Read the model definition and answer for the solid it produces. Units are mm, in the model's axes. A direction names the side the tool comes from. Coordinates: 2 decimals unless noted, no trailing zeros. Write each loop counter-clockwise with the first axis right and the second up, starting at its lowest first coordinate (ties: lowest second). Pieces come first, ordered by that corner, then holes. Notation, with made-up numbers: (-1.5, -1) - (51.5, -1) arc R18 cw to (51.5, 29) - close; hole circle Ø11 at (84.5, 48.5). An arc over 180 degrees is marked (long way). Return JSON: item names as keys, results as strings.
```python
from build123d import *

# Parameters (mm, degrees)
BOSS_EXTRUDE1_DEPTH = 34
CUT_EXTRUDE2_START  = -2.320517
SKETCH3_R           = 1.1
CUT_EXTRUDE2_DEPTH  = 2.320517
SKETCH4_R           = 2
CUT_EXTRUDE3_DEPTH  = 1
FILLET1_R           = 2


with BuildPart() as part:
    # Sketch1 → Boss-Extrude1 (new body)
    with BuildSketch(Plane.XY):
        with BuildLine():
            Line((0.25, 38.599190406), (0.25, 41.099190406))
            Line((0.25, 41.099190406), (8.207138981, 40.272184219))
            ThreePointArc((8.207138981, 40.272184219), (8.347930101, 39.521941532), (8.972631806, 39.083268523))
            ThreePointArc((8.972631806, 39.083268523), (0, -40.1), (-8.972631806, 39.083268523))
            ThreePointArc((-8.972631806, 39.083268523), (-8.347930101, 39.521941532), (-8.207138981, 40.272184219))
            Line((-8.207138981, 40.272184219), (-0.25, 41.099190406))
            Line((-0.25, 41.099190406), (-0.25, 38.599190406))
            ThreePointArc((-0.25, 38.599190406), (0, -38.6), (0.25, 38.599190406))
        make_face()
    extrude(amount=BOSS_EXTRUDE1_DEPTH)

    # Sketch3 → Cut-Extrude2 (cut)
    with BuildSketch(Plane(origin=(-4.228569491, 40.685687313, 0), x_dir=(0.994642373, 0.103375773, 0), z_dir=(-0.103375773, 0.994642373, 0)).offset(CUT_EXTRUDE2_START)):
        with Locations((0, -4)):
            Circle(SKETCH3_R)
        with Locations((0, -30)):
            Circle(SKETCH3_R)
    cut_extrude2 = extrude(amount=CUT_EXTRUDE2_DEPTH, mode=Mode.SUBTRACT)

    # Sketch4 → Cut-Extrude3 (cut)
    with BuildSketch(Plane(origin=(-4.228569491, 40.685687313, 0), x_dir=(0.994642373, 0.103375773, 0), z_dir=(-0.103375773, 0.994642373, 0))):
        with Locations((0, -4)):
            Circle(SKETCH4_R)
        with Locations((0, -30)):
            Circle(SKETCH4_R)
    cut_extrude3 = extrude(amount=-CUT_EXTRUDE3_DEPTH, mode=Mode.SUBTRACT)

    # Mirror3: Cut-Extrude2, Cut-Extrude3 across plane
    add(cut_extrude2.mirror(Plane(origin=(0, 0, 0), x_dir=(0, 0, 1), z_dir=(1, 0, 0))), mode=Mode.SUBTRACT)
    add(cut_extrude3.mirror(Plane(origin=(0, 0, 0), x_dir=(0, 0, 1), z_dir=(1, 0, 0))), mode=Mode.SUBTRACT)

    # Fillet1
    fillet1_edges = [part.edges().sort_by_distance(p)[0] for p in [
        (-0.25, 39.849190406, 0),
        (0.25, 39.849190406, 34),
        (0.25, 39.849190406, 0),
        (-0.25, 39.849190406, 34),
    ]]
    fillet(fillet1_edges, radius=FILLET1_R)


solid = part.part
```
(1) A cutting plane is placed at B-B (z = 22). Determine the outline of the cut face in (x, y), and give its area (3 significant figures).
Answer:
{"outline": "(-8.97, 39.08) arc R40.1 ccw (long way) to (8.97, 39.08) arc R1.01 cw to (8.21, 40.27) - (0.25, 41.1) - (0.25, 38.6) arc R38.6 cw (long way) to (-0.25, 38.6) - (-0.25, 41.1) - (-8.21, 40.27) arc R1.01 cw to start", "area": "384 mm²"}
(2) Determine the mould class of faces 1 (the face through (0.82, 39.83, 0.6)), 2 (the face through (-4.15, 39.69, 31.31)), 3 (the face through (1.637, -40.067, 16.762)), 4 (the face through (39, 1, 34)) for opening direction X: +X half, -X half, draft (parallel to the pull), parting line (faces both ways), or undercut.
Answer:
{"face 1": "undercut", "face 2": "undercut", "face 3": "parting line", "face 4": "draft"}
(3) A cutting plane is placed at A-A (y = 0). Determine the outline of the cut face in (x, z).
Answer:
{"outline": "(-40.1, 0) - (-38.6, 0) - (-38.6, 34) - (-40.1, 34) - close; (38.6, 0) - (40.1, 0) - (40.1, 34) - (38.6, 34) - close"}
(4) Straight lines are drawn through the part: line 1 (X direction, y = 0, z = 23); line 2 (X direction, y = 16, z = 32.5); line 3 (Y direction, x = 32, z = 26). For each, find the intervals that lie inside material, in ascending order. Write a range as from..to.
Answer:
{"line 1": "-40.1..-38.6, 38.6..40.1", "line 2": "-36.77..-35.13, 35.13..36.77", "line 3": "-24.17..-21.59, 21.59..24.17"}
(5) A cutting plane is placed at C-C (y = 11). Determine the outline of the cut face in (x, z).
Answer:
{"outline": "(-38.56, 0) - (-37, 0) - (-37, 34) - (-38.56, 34) - close; (37, 0) - (38.56, 0) - (38.56, 34) - (37, 34) - close"}
(6) Flat-ended cylindrical pins translate along their axes: P1, Ø8, axis at x = 6, z = 28.5, coming from the -Y side; P2, Ø10, axis at y = 27, z = 7, coming from the -X side; P3, Ø3, axis at x = -22.5, z = 19.5, coming from the +Y side. Find the tip coordinate at first contact, or state that the pin passes through.
Answer:
{"P1": "y = -40.05", "P2": "x = -33.53", "P3": "y = 34.16"}
(7) Which of the six approach directions +Z, -Z, +X, -X, +Y, -Y give full straight-line access (tool end or side, diameter ignored) to faces 5 (the face through (-1.694, -38.563, 16.762)), 6 (the face through (0.82, 39.83, 33.4)), 7 (the face through (-0.85, 39.8, 0.57)), 8 (the face through (0.25, 40, 17))?
Answer:
{"face 5": "+Z, -Z", "face 6": "+Z, +Y", "face 7": "-Z, +Y", "face 8": "+Z, -Z, +Y"}
